```python
from build123d import *

# Parameters (mm, degrees)
SKETCH268_R     = 4
PAD107_DEPTH    = 10
SKETCH269_R     = 4
SKETCH269_R_2   = 2.1
PAD108_DEPTH    = 2
SKETCH270_R     = 1.5
POCKET131_DEPTH = 4.001


with BuildPart() as part:
    # Sketch268 → Pad107 (new body)
    with BuildSketch(Plane.XY):
        Circle(SKETCH268_R)
        with BuildLine():
            Line((-1.360147, 1.6), (1.360147, 1.6))
            ThreePointArc((-1.360147, 1.6), (0, -2.1), (1.360147, 1.6))
        make_face(mode=Mode.SUBTRACT)
    extrude(amount=PAD107_DEPTH)

    # Sketch269 (on Face5 of Pad107) → Pad108 (join)
    with BuildSketch(Plane.XY.offset(10)):
        Circle(SKETCH269_R)
        Circle(SKETCH269_R_2, mode=Mode.SUBTRACT)
    extrude(amount=PAD108_DEPTH)

    # Sketch270 → Pocket131 (cut, through all)
    with BuildSketch(Plane.XZ):
        with Locations((0, 3)):
            Circle(SKETCH270_R)
    extrude(amount=-POCKET131_DEPTH, mode=Mode.SUBTRACT)


solid = part.part
```
Build history of the part. All positions in model axes, mm. A direction names the side the tool comes from. Coordinates: 2 decimals unless noted, no trailing zeros. Write each loop counter-clockwise with the first axis right and the second up, starting at its lowest first coordinate (ties: lowest second). Pieces come first, ordered by that corner, then holes.
1. Band-saw the part on A-A, the plane x = 0. Give the cut face in (y, z).
Answer block:
outline: (-4, 0) - (-2.1, 0) - (-2.1, 12) - (-4, 12) - close; (1.6, 0) - (4, 0) - (4, 1.5) - (1.6, 1.5) - close; (1.6, 4.5) - (4, 4.5) - (4, 12) - (2.1, 12) - (2.1, 10) - (1.6, 10) - close
2. 3-axis set-ups, long thin cutter, end or side, ignore diameter. For faces 1 (the flat face through (0, 1.6, 1)), 2 (the flat face through (2, -2, 12)): which of +Z, -Z, +X, -X, +Y, -Y reach the whole face in a straight line?
Answer block:
face 1: +Z, -Z
face 2: +Z, +X, -X, +Y, -Y
3. Pull direction Y, two halves, no side cores. Call faces 3 (the flat face through (0, 1.6, 7)), 4 (the cylindrical face through (1.43, 2.72, 3.45)), 5 (the cylindrical face through (-0.867, -3.905, 5.916)): released by +Y, released by -Y, zero draft, split by the parting line, or undercut.
Answer block:
face 3: undercut
face 4: zero draft
face 5: split by the parting line
4. Band-saw the part on B-B, the plane y = 0. Give the cut face in (x, z).
Answer block:
outline: (-4, 0) - (-2.1, 0) - (-2.1, 12) - (-4, 12) - close; (2.1, 0) - (4, 0) - (4, 12) - (2.1, 12) - close
5. Band-saw the part on D-D, the plane z = 1.75. Give the cut face in (x, y), and give its area (3 significant figures).
Answer block:
outline: (-1.36, 1.6) - (-0.83, 1.6) - (-0.83, 3.91) arc R4 ccw (long way) to (0.83, 3.91) - (0.83, 1.6) - (1.36, 1.6) arc R2.1 cw (long way) to start
area: 33.4 mm2
6. Band-saw the part on C-C, the plane z = 7.5. Give the cut face in (x, y).
Answer block:
outline: circle Ø8 at (0, 0); hole (-1.36, 1.6) arc R2.1 ccw (long way) to (1.36, 1.6) - close
7. Drill centre lines: probe 1 along Y at (x, z) = (0, 8.25); probe 2 along Z at (x, y) = (0, 2.9); probe 3 along Z at (x, y) = (0, 2.05). Where is each one in solid material? Low to high.
Answer block:
probe 1: y = -4 to -2.1, 1.6 to 4
probe 2: z = 0 to 1.5, 4.5 to 12
probe 3: z = 0 to 1.5, 4.5 to 10
